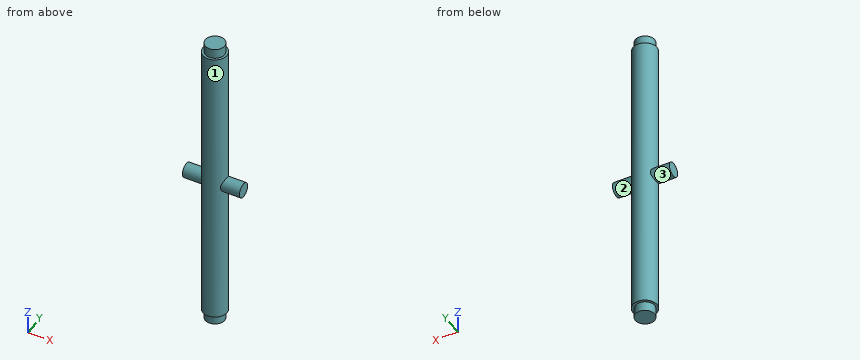
Autodesk Fusion 360 part; units mm, degrees
sketch "Sketch8" plane through (0, 0, 0) normal (0, 0, 1) x (1, 0, 0)
  circle A0 centre (0, 0) radius 15
  circle A1 centre (0, 0) radius 25
  dimension "d21" = 30
  dimension "d22" = 50
extrude "Extrude3" add sketch "Sketch8" along normal mid plane 600 makes body 1
sketch "Sketch9" plane through (0, 0, 0) normal (1, 0, 0) x (0, 0, -1)
  circle A0 centre (0, 0) radius 10
  circle A1 centre (0, 0) radius 15
  dimension "d25" = 20
  dimension "d26" = 30
extrude "Extrude4" cut sketch "Sketch9" along normal mid plane 100 contours A0 bodies 1
extrude "Extrude5" add sketch "Sketch9" along normal mid plane 100 separate body makes body 2
extrude "Extrude6" cut sketch "Sketch8" along normal mid plane 600 contours A0 bodies 2
combine "Combine1" operation add target body 1 tool bodies 2
sketch "Sketch10" plane through (0, 0, -300) normal (0, 0, -1) x (-1, 0, 0)
  circle A0 centre (0, 0) radius 15
  circle A1 centre (0, 0) radius 25
  circle A2 centre (0, 0) radius 15
  circle A3 centre (0, 0) radius 20
  dimension "d33" = 30
  dimension "d34" = 40
extrude "Extrude7" add sketch "Sketch10" along normal blind 10 contours A3 bodies 1
sketch "Sketch11" plane through (0, 0, 300) normal (0, 0, 1) x (1, 0, 0)
  circle A0 centre (0, 0) radius 15
  circle A1 centre (0, 0) radius 25
  circle A2 centre (0, 0) radius 15
  circle A3 centre (0, 0) radius 20
  dimension "d38" = 30
  dimension "d39" = 40
extrude "Extrude8" add sketch "Sketch11" along normal blind 10 contours A3 bodies 1
sketch "Sketch12" plane through (0, 0, -310) normal (0, 0, -1) x (-1, 0, 0)
  circle A0 centre (0, 0) radius 15
  circle A1 centre (0, 0) radius 20
  circle A2 centre (0, 0) radius 20
  dimension "d42" = 40
extrude "Extrude9" add sketch "Sketch12" along normal blind 10 contours A0 | A1 A2 bodies 1
sketch "Sketch13" plane through (0, 0, 310) normal (0, 0, 1) x (1, 0, 0)
  circle A0 centre (0, 0) radius 15
  circle A1 centre (0, 0) radius 20
  circle A2 centre (0, 0) radius 20
  dimension "d45" = 40
extrude "Extrude10" add sketch "Sketch13" along normal blind 10 contours A0 | A1 A2 bodies 1
sketch "Sketch14" plane through (-50, 0, 0) normal (-1, 0, 0) x (0, 0, 1)
  circle A0 centre (0, 0) radius 10
  circle A1 centre (0, 0) radius 15
  circle A2 centre (0, 0) radius 15
  dimension "d48" = 30
extrude "Extrude11" add sketch "Sketch14" along normal blind 10 contours A0 | A1 A2 bodies 1
sketch "Sketch15" plane through (50, 0, 0) normal (1, 0, 0) x (0, 0, -1)
  circle A0 centre (0, 0) radius 10
  circle A1 centre (0, 0) radius 15
  circle A2 centre (0, 0) radius 15
  dimension "d51" = 30
extrude "Extrude12" add sketch "Sketch15" along normal blind 10 contours A0 | A1 A2 bodies 1
equation "LC_id = 30 mm"
equation "LC_od = 50 mm"
equation "SC_id = 20 mm"
equation "SC_od = 30 mm"
equation "LC_l = 300 mm"
equation "SC_l = 50 mm"
equation "SC_c = LC_l / 2.0"
equation "LC_w_id = LC_id"
equation "LC_w_od = 1.0 / 2.0 * ( LC_od + LC_id )"
equation "d21 = LC_id"
equation "d22 = LC_od"
equation "d23 = LC_l"
equation "d25 = SC_id"
equation "d26 = SC_od"
equation "d27 = SC_l"
equation "d29 = SC_l"
equation "d31 = LC_l"
equation "d33 = LC_w_id"
equation "d34 = LC_w_od"
equation "LC_w_l = 10 mm"
equation "d36 = LC_w_l"
equation "d38 = LC_w_id"
equation "d39 = LC_w_od"
equation "d40 = LC_w_l"
equation "d42 = LC_w_od"
equation "d45 = LC_w_od"
equation "d48 = SC_od"
equation "d51 = SC_od"
properties part number "Configuration 3"
Geometry check sheet. Reference: the model listing, model coordinates, mm. Face numbers are marked on the shaded views. A direction names the side the tool comes from. Coordinates: 2 decimals unless noted, no trailing zeros. Write each loop counter-clockwise with the first axis right and the second up, starting at its lowest first coordinate (ties: lowest second). Pieces come first, ordered by that corner, then holes. Notation, with made-up numbers: M 55.25,58.25 L 96.25,58.25 A8 ccw 96.25,62.25 Z; hole C -38,7 d5. An arc over 180 degrees is marked long. One line per item, written item: value. Start each with the question number.
(1) Tool access check on the marked faces 1, 2 and 3. Record the directions out of +Z, -Z, +X, -X, +Y, -Y that give a thin tool (end or side, any length) a straight path to the whole face; none if there is none.
(2) Depth check by flat-ended pin: pin 1 (12 mm diameter, centred on x = -1.5, z = -241, fed in from +Y); pin 2 (2 mm diameter, centred on x = 44, y = -1.5, fed in from -Z); pin 3 (10 mm diameter, centred on y = -2.5, z = -102.5, fed in from -X); pin 4 (1.5 mm diameter, centred on x = -26.5, z = 196, fed in from +Y). Enter the tip coordinate at first touch or a pass-through.
(3) Sectioned sample at B-B, the plane x = 0. Enter the section's corners in (y, z), and give its area (3 significant figures).
(4) Scan lines: line 1 along Y through (x, z) = (0, -303); line 2 along Y through (x, z) = (40.5, 0); line 3 along Z through (x, y) = (22.25, 0). Record each from-to range of solid material in increasing order. Write a range as [from, to].
(5) Sectioned sample at D-D, the plane z = -276.5. Enter the section's corners in (x, y), and give its area (3 significant figures).
(6) Sectioned sample at A-A, the plane z = 0. Enter the section's corners in (x, y), and give its area (3 significant figures).
Filled sheet:
1. face 1: none
1. face 2: +X
1. face 3: -X
2. pin 1: y = 25
2. pin 2: z = -14.99
2. pin 3: x = -25
2. pin 4: through
3. outline: M -25,-300 L -20,-300 L -20,-320 L 20,-320 L 20,-300 L 25,-300 L 25,300 L 20,300 L 20,320 L -20,320 L -20,300 L -25,300 Z; hole M -15,-310 L 15,-310 L 15,310 L -15,310 Z
3. area: 13,000 mm²
4. line 1: [-20, -15], [15, 20]
4. line 2: [-15, -10], [10, 15]
4. line 3: [-300, -10], [10, 300]
5. outline: C 0,0 d50; hole C 0,0 d30
5. area: 1,260 mm²
6. outline: M -60,-15 L -20,-15 A25 ccw 20,-15 L 60,-15 L 60,15 L 20,15 A25 ccw -20,15 L -60,15 Z; hole M -50,-10 L -11.18,-10 A15 ccw 11.18,-10 L 50,-10 L 50,10 L 11.18,10 A15 ccw -11.18,10 L -50,10 Z
6. area: 2,000 mm²
